Print and shaded views of the part. All mm, measured from the part's lowest x, y and z. Coordinates: 2 decimals unless noted, no trailing zeros. Order: outer loops, then holes, each group sorted by start corner. A loop starts at its lowest first (then second) coordinate and runs counter-clockwise, first axis right, second up. Notation, with made-up numbers: (20, 9) -> (46, 9) arc R8 cw to (46, 24) -> close; hole circle Ø1 at (61, 33). An arc over 180 degrees is marked (long way). Return JSON: item names as keys, results as strings. Group by question number.
1) Pull direction Y, two halves, no side cores. Call the marked faces 1, 2 and 3: +Y half, -Y half, draft (parallel to the pull), parting line (faces both ways), or undercut.
2) Cut at B-B (y = 3.5). Write the cut outline in (x, z), and give its area (3 significant figures).
3) Probe line 1 (Y direction, x = 19, z = 4.8) (1 decimal); line 2 (Y direction, x = 19, z = 1.5) (1 decimal); line 3 (Y direction, x = 8.5, z = 0.75) (1 decimal). List the from-to ranges inside material, lowest first.
4) Flat gauge pins, fed straight in: pin 1 (2.5 mm diameter, centred on x = 19, y = 4.29, fed in from +Z); pin 2 (1.5 mm diameter, centred on x = 19.5, y = 5.5, fed in from -Z); pin 3 (1 mm diameter, centred on x = 26, z = 4.5, fed in from -Y) (1 decimal). Where does each tip first touch, or does it go through?
5) Cut at C-C (z = 6.25). Write the cut outline in (x, y) (1 decimal).
6) Cut at A-A (x = 19). Write the cut outline in (y, z).
7) Cut at D-D (y = 6.25). Write the cut outline in (x, z) (1 decimal).
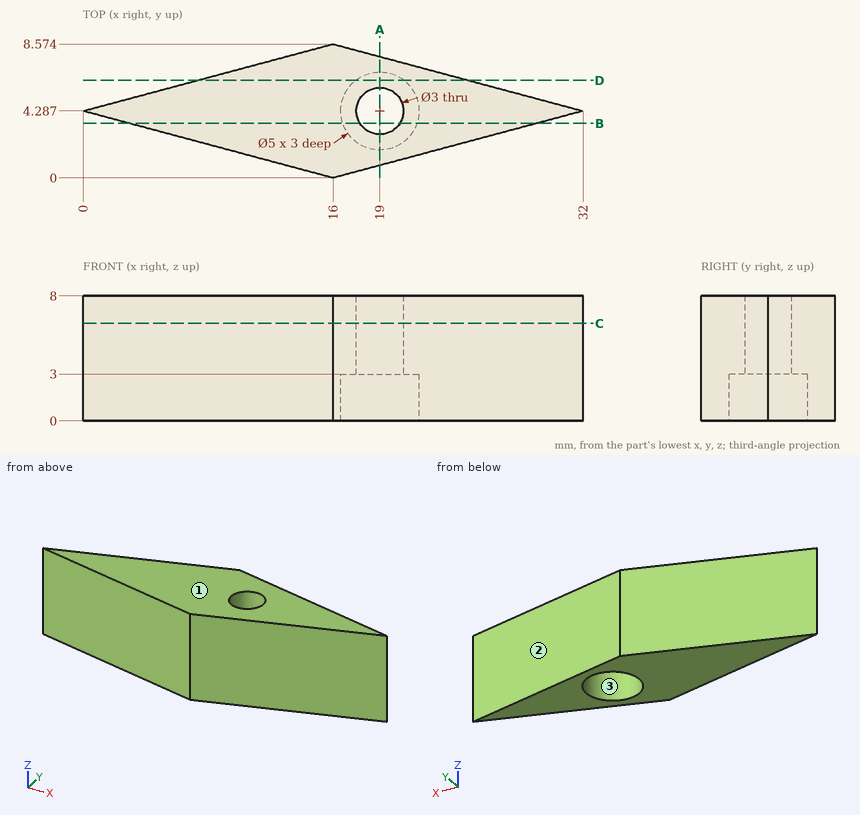
Answers below:
{
 "1": {"face 1": "draft", "face 2": "+Y half", "face 3": "undercut"},
 "2": {"outline": "(2.94, 0) -> (16.63, 0) -> (16.63, 3) -> (17.72, 3) -> (17.72, 8) -> (2.94, 8) -> close; (20.28, 3) -> (21.37, 3) -> (21.37, 0) -> (29.06, 0) -> (29.06, 8) -> (20.28, 8) -> close", "area": "182 mm^2"},
 "3": {"line 1": "y = 0.8 to 2.8, 5.8 to 7.8", "line 2": "y = 0.8 to 1.8, 6.8 to 7.8", "line 3": "y = 2 to 6.6"},
 "4": {"pin 1": "passes through", "pin 2": "stops at z = 3", "pin 3": "stops at y = 2.5"},
 "5": {"outline": "(0, 4.3) -> (16, 0) -> (32, 4.3) -> (16, 8.6) -> close; hole circle Ø3 at (19, 4.3)"},
 "6": {"outline": "(0.8, 0) -> (1.79, 0) -> (1.79, 3) -> (2.79, 3) -> (2.79, 8) -> (0.8, 8) -> close; (5.79, 3) -> (6.79, 3) -> (6.79, 0) -> (7.77, 0) -> (7.77, 8) -> (5.79, 8) -> close"},
 "7": {"outline": "(7.3, 0) -> (17.5, 0) -> (17.5, 3) -> (20.5, 3) -> (20.5, 0) -> (24.7, 0) -> (24.7, 8) -> (7.3, 8) -> close"}
}
